from build123d import *

# Parameters (mm, degrees)
SKETCH1_R           = 8
SKETCH1_R_2         = 3.05
BOSS_EXTRUDE1_DEPTH = 1.625
SKETCH3_R           = 3.5
SKETCH3_R_2         = 2
BOSS_EXTRUDE2_DEPTH = 0.75
SKETCH4_R           = 6.5
SKETCH4_R_2         = 3
CUT_EXTRUDE1_DEPTH  = 0.5
FILLET1_R           = 0.5


with BuildPart() as part:
    # Sketch1 → Boss-Extrude1 (new, symmetric)
    with BuildSketch(Plane(origin=(0, 0, 0), x_dir=(1, 0, 0), z_dir=(0, 1, 0))):
        with Locations(Location((0, 0, 0), (0, 0, 90))):
            Circle(SKETCH1_R)
        with Locations(Location((0, 0, 0), (0, 0, 90))):
            Circle(SKETCH1_R_2, mode=Mode.SUBTRACT)
    extrude(amount=BOSS_EXTRUDE1_DEPTH, both=True)

    # Sketch2 → Cut-Revolve1 (revolve, cut)
    with BuildSketch(Plane(origin=(0, 0, 0), x_dir=(0, 0, -1), z_dir=(1, 0, 0)), mode=Mode.PRIVATE) as cut_revolve1_sk:
        with BuildLine():
            Line((-8, 0.75), (-8, -0.75))
            ThreePointArc((-8, -0.75), (-7.25, 0), (-8, 0.75))
        make_face()
    revolve(cut_revolve1_sk.sketch.rotate(Axis((0, 1.625, 0), (0, -1, 0)), 180), axis=Axis((0, 1.625, 0), (0, -1, 0)), mode=Mode.SUBTRACT)

    # Sketch3 → Boss-Extrude2 (add)
    with BuildSketch(Plane(origin=(0, 1.625, 0), x_dir=(1, 0, 0), z_dir=(0, 1, 0))):
        Circle(SKETCH3_R)
        with Locations(Location((0, 0, 0), (0, 0, 270))):
            Circle(SKETCH3_R_2, mode=Mode.SUBTRACT)
    extrude(amount=-BOSS_EXTRUDE2_DEPTH)

    # Sketch4 → Cut-Extrude1 (cut)
    with BuildSketch(Plane.XZ.offset(1.625)):
        with Locations(Location((0, 0, 0), (0, 0, 270))):
            Circle(SKETCH4_R)
        Circle(SKETCH4_R_2, mode=Mode.SUBTRACT)
    extrude(amount=-CUT_EXTRUDE1_DEPTH, mode=Mode.SUBTRACT)

    # Fillet1
    fillet1_edges = [part.edges().sort_by_distance(p)[0] for p in [
        (0, 0.875, 3.05),
        (0, -1.125, 3.05),
    ]]
    fillet(fillet1_edges, radius=FILLET1_R)


solid = part.part
Build history of the part. All positions in model axes, mm. A direction names the side the tool comes from. Give positions to 0.01 mm unless a question says otherwise; leave off trailing zeros. Loops run counter-clockwise (first coordinate to the right, second up) from the corner with the lowest first, then second, coordinate; pieces in that order, holes last. Notation, with made-up numbers: (-26, 15) - (-22, 15) arc R10 cw to (-22, 22) - close; hole circle Ø10 at (26, 81.5). An arc over 180 degrees is marked (long way). Write item = value, one per line. Start each with the question number.
1) Band-saw the part on B-B on x = 0. Give the cut face in (y, z) (3 decimals).
2) Band-saw the part on C-C on y = 0.1. Give the cut face in (x, z), plus the area to 3 significant figures.
3) Drop flat-ended pins along their axis: pin 1 Ø1 at (x, y) = (1.5, 1) entering from -Z; pin 2 Ø4.5 at (x, z) = (0, 0) entering from -Y (3 decimals); pin 3 Ø1.5 at (y, z) = (-0.5, 5) entering from -X. Give the stop position or say it passes through.
4) Band-saw the part on A-A on z = 0. Give the cut face in (x, y) (3 decimals).
5) Pull direction Z, two halves, no side cores. Call faces 1 (the cylindrical face through (7.81, 1.19, 1.73)), 2 (the flat face through (2, 1.625, -2)), 3 (the cylindrical face through (1.856, -0.132, 2.42)): +Z half, -Z half, draft (parallel to the pull), parting line (faces both ways), or undercut.
6) Probe probe 1 along X at (y, z) = (1.3, 0); probe 2 along X at (y, z) = (-1.2, 0); probe 3 along Y at (x, z) = (3.5, -4.75) (3 decimals). List the from-to ranges inside material, lowest first. Write a range as from..to.
7) Tool access for faces 4 (the cylindrical face through (-3.955, -1.378, 5.158)), 5 (the flat face through (-7, -1.625, 0)): list every direction of +Z, -Z, +X, -X, +Y, -Y with a clear straight run to the whole face (end or side of a thin tool).
Final values:
q1.outline = (-1.625, -8) - (-0.75, -8) arc R0.75 cw to (0.75, -8) - (1.625, -8) - (1.625, -2) - (0.875, -2) - (0.875, -2.55) arc R0.5 cw to (0.375, -3.05) - (-0.625, -3.05) arc R0.5 ccw to (-1.125, -3.55) - (-1.125, -6.5) - (-1.625, -6.5) - close; (-1.625, 6.5) - (-1.125, 6.5) - (-1.125, 3.55) arc R0.5 ccw to (-0.625, 3.05) - (0.375, 3.05) arc R0.5 cw to (0.875, 2.55) - (0.875, 2) - (1.625, 2) - (1.625, 8) - (0.75, 8) arc R0.75 cw to (-0.75, 8) - (-1.625, 8) - close
q2.outline = circle Ø14.51 at (0, 0); hole circle Ø6.1 at (0, 0)
q2.area = 136 mm²
q3.pin_1 = -7.94
q3.pin_2 = 0.875
q3.pin_3 = -6.75
q4.outline = (-8, -1.625) - (-6.5, -1.625) - (-6.5, -1.125) - (-3.55, -1.125) arc R0.5 ccw to (-3.05, -0.625) - (-3.05, 0.375) arc R0.5 cw to (-2.55, 0.875) - (-2, 0.875) - (-2, 1.625) - (-8, 1.625) - (-8, 0.75) arc R0.75 cw to (-8, -0.75) - close; (2, 0.875) - (2.55, 0.875) arc R0.5 cw to (3.05, 0.375) - (3.05, -0.625) arc R0.5 ccw to (3.55, -1.125) - (6.5, -1.125) - (6.5, -1.625) - (8, -1.625) - (8, -0.75) arc R0.75 cw to (8, 0.75) - (8, 1.625) - (2, 1.625) - close
q5.face_1 = parting line
q5.face_2 = draft
q5.face_3 = undercut
q6.probe_1 = -8..-2, 2..8
q6.probe_2 = -8..-6.5, 6.5..8
q6.probe_3 = -1.125..1.625
q7.face_4 = -Y
q7.face_5 = +Z, -Z, +X, -X, -Y
